The listing builds one solid part. Answer for the finished solid, in the listing's coordinates (mm). Face numbers are marked on the shaded views. A direction names the side the tool comes from. Round coordinates to 2 decimals unless told otherwise and drop trailing zeros. Order: outer loops, then holes, each group sorted by start corner. A loop starts at its lowest first (then second) coordinate and runs counter-clockwise, first axis right, second up. Notation, with made-up numbers: (-4, 14.5) - (55, 14.5) arc R35 ccw to (55, 52.5) - close; hole circle Ø6 at (47.25, 17.25). An arc over 180 degrees is marked (long way). One line per item, written item: value. Start each with the question number.
1. For a pull along Y with two mould halves and no side action, classify the marked faces 1, 2 and 3 as released by +Y, released by -Y, zero draft, split by the parting line, or undercut.
2. Section B-B, the plane y = 14 is taken. Give the vertices of the cut face in (x, z), then the cut area to 3 significant figures.
3. Section C-C, the plane x = 0.5 is taken. Give the vertices of the cut face in (y, z), then the cut area to 3 significant figures.
4. Straight lines are drawn through the part: line 1 (X direction, y = 7, z = 8.75); line 2 (X direction, y = 6, z = 8.75); line 3 (X direction, y = -3, z = 7.25). For each, find the intervals that lie inside material, in ascending order.
5. Section A-A, the plane z = 4 is taken. Give the vertices of the cut face in (x, y).
6. Flat-ended cylindrical pins translate along their axes: P1, Ø2, axis at y = 14.5, z = 2, coming from the +X side; P2, Ø1, axis at x = -3, z = 5, coming from the +Y side; P3, Ø1, axis at x = -9.5, z = 5, coming from the -Y side; P4, Ø16, axis at x = -14.13, y = 5.38, coming from the +Z side. Find the tip coordinate at first contact, or state that the pin passes through.
7. A tool of negligible diameter and unlimited length cuts with its end or side. For the marked faces 4 and 5, from which of +Z, -Z, +X, -X, +Y, -Y can it reach the whole face along a straight path? Write none if from no direction.
8. Section D-D, the plane x = -12.5 is taken. Give the vertices of the cut face in (y, z).
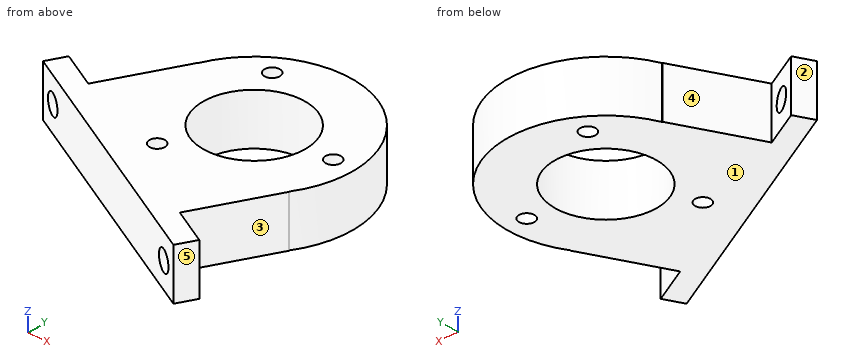
from build123d import *

# Parameters (mm, degrees)
SKETCH1_R           = 19.3
SKETCH1_R_2         = 10
SKETCH1_R_3         = 1.5
BOSS_EXTRUDE1_DEPTH = 10
SKETCH2_W           = 55
SKETCH2_H           = 10
BOSS_EXTRUDE2_DEPTH = 50
CUT_EXTRUDE1_DEPTH  = 50
SKETCH5_R           = 2
CUT_EXTRUDE2_DEPTH  = 50
SKETCH1_2_R         = 10
SKETCH1_2_R_2       = 1.5
CUT_EXTRUDE3_DEPTH  = 50


with BuildPart() as part:
    # Sketch1 → Boss-Extrude1 (new body)
    with BuildSketch(Plane.XY):
        with Locations((-14.127422454, 5.37928778)):
            Circle(SKETCH1_R)
        with Locations((-14.127422454, 5.37928778)):
            Circle(SKETCH1_R_2, mode=Mode.SUBTRACT)
        with Locations((0.862954929, 5.91648973)):
            Circle(SKETCH1_R_3, mode=Mode.SUBTRACT)
        with Locations((-22.08784168, 18.092734431)):
            Circle(SKETCH1_R_3, mode=Mode.SUBTRACT)
        with Locations((-21.15738061, -7.87136082)):
            Circle(SKETCH1_R_3, mode=Mode.SUBTRACT)
    extrude(amount=BOSS_EXTRUDE1_DEPTH)

    # Sketch2 → Boss-Extrude2 (add)
    with BuildSketch(Plane(origin=(-14.175728754, -26.918620376, 0), x_dir=(0.8848093624477475, -0.46595320808511503, 0), z_dir=(-0.46595320808511503, -0.8848093624477475, 0))):
        with Locations((-15.006572053, 5)):
            Rectangle(SKETCH2_W, SKETCH2_H)
    extrude(amount=-BOSS_EXTRUDE2_DEPTH)

    # Sketch4 → Cut-Extrude1 (cut)
    with BuildSketch(Plane(origin=(0, 0, 0), x_dir=(-1, 0, 0), z_dir=(0, 0, -1))):
        with BuildLine():
            Line((-20.176233667, 11.500494914), (-9.425814966, -8.913724692))
            Line((-9.425814966, -8.913724692), (-2.170378194, -5.092908386))
            Line((-2.170378194, -5.092908386), (-2.106184539, -5.059103093))
            ThreePointArc((-2.106184539, -5.059103093), (5.134525538, 22.456108476), (31.919069541, 12.859080153))
            Line((31.919069541, 12.859080153), (31.983263196, 12.892885446))
            Line((31.983263196, 12.892885446), (39.238699968, 16.713701752))
            Line((39.238699968, 16.713701752), (28.488281268, 37.127921359))
            Line((28.488281268, 37.127921359), (-20.176233667, 11.500494914))
        make_face()
        Polygon((47.126409591, 1.735546861), (39.238699968, 16.713701752), (31.983263196, 12.892885446), (39.870972819, -2.085269445), align=None)
        Polygon((-2.170378194, -5.092908386), (-9.425814966, -8.913724692), (-1.538105343, -23.891879583), (5.717331429, -20.071063277), align=None)
        Polygon((48.990222424, -1.803690589), (0.325707489, -27.431117033), (3.121426738, -32.739973208), (51.785941672, -7.112546763), align=None)
    extrude(amount=-CUT_EXTRUDE1_DEPTH, mode=Mode.SUBTRACT)

    # Sketch5 → Cut-Extrude2 (cut)
    with BuildSketch(Plane(origin=(-9.516196674, -18.070526751, 0), x_dir=(0.8848093624477471, -0.4659532080851159, 0), z_dir=(0.4659532080851159, 0.8848093624477471, 0))):
        with Locations(Location((-38.406572053, -5, 0), (0, 0, 180))):
            Circle(SKETCH5_R)
        with Locations(Location((8.393427947, -5, 0), (0, 0, 180))):
            Circle(SKETCH5_R)
    extrude(amount=-CUT_EXTRUDE2_DEPTH, mode=Mode.SUBTRACT)

    # Sketch1_2 → Cut-Extrude3 (cut)
    with BuildSketch(Plane.XY):
        with Locations((-14.127422454, 5.37928778)):
            Circle(SKETCH1_2_R)
        with Locations((-21.15738061, -7.87136082)):
            Circle(SKETCH1_2_R_2)
        with Locations((-22.08784168, 18.092734431)):
            Circle(SKETCH1_2_R_2)
        with Locations((0.862954929, 5.91648973)):
            Circle(SKETCH1_2_R_2)
    extrude(amount=CUT_EXTRUDE3_DEPTH, mode=Mode.SUBTRACT)


solid = part.part
Answer list:
1. face 1: zero draft
1. face 2: released by +Y
1. face 3: undercut
2. outline: (-31.4, 0) - (-19.2, 0) - (-19.2, 10) - (-31.4, 10) - close; (-9.06, 0) - (3.14, 0) - (3.14, 10) - (-9.06, 10) - close
2. area: 244 mm²
3. outline: (-25.86, 0) - (-23.35, 0) - (-23.35, 10) - (-25.86, 10) - close; (-8.26, 0) - (4.46, 0) - (4.46, 10) - (-8.26, 10) - close; (7.37, 0) - (17.97, 0) - (17.97, 10) - (7.37, 10) - close
3. area: 258 mm²
4. line 1: x = -35.09 to -24, -4.26 to -0.17, 1.9 to 5.1
4. line 2: x = -35.61 to -24.11, -4.15 to -0.63, 2.36 to 5.16
4. line 3: x = -46.72 to -19.59, -8.67 to 3.26
5. outline: (-48.99, -1.8) - (-46.9, -2.91) - (-45.03, 0.63) - (-47.13, 1.74) - close; (-43.83, -4.52) - (-5.49, -24.71) - (-3.62, -21.17) - (-5.72, -20.07) - (2.17, -5.09) - (2.11, -5.06) arc R19.3 ccw (long way) to (-31.92, 12.86) - (-31.98, 12.89) - (-39.87, -2.09) - (-41.97, -0.98) - close; (-2.42, -26.33) - (-0.33, -27.43) - (1.54, -23.89) - (-0.56, -22.79) - close; hole circle Ø20 at (-14.13, 5.38); hole circle Ø3 at (-22.09, 18.09); hole circle Ø3 at (-21.16, -7.87); hole circle Ø3 at (0.86, 5.92)
6. P1: stops at x = 3.38
6. P2: stops at y = 21.49
6. P3: stops at y = -22.86
6. P4: passes through
7. face 4: +Z, -Z, +Y
7. face 5: +Z, -Z, +X, -Y
8. outline: (-21.02, 0) - (-4.49, 0) - (-4.49, 10) - (-21.02, 10) - close; (15.25, 0) - (24.61, 0) - (24.61, 10) - (15.25, 10) - close
